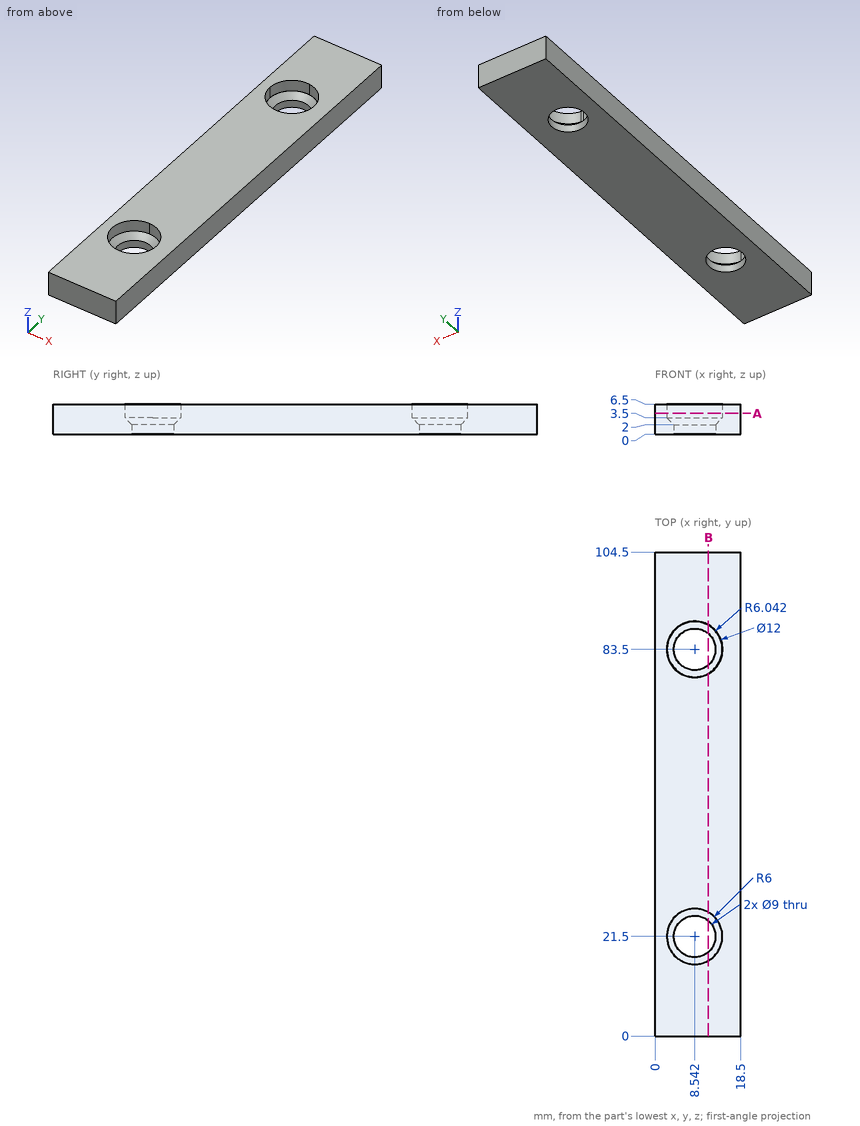
Could you check a few things on this drawing? It's one solid part, dimensions in mm from its lowest x, y, z. Round coordinates to 2 decimals unless told otherwise and drop trailing zeros. Write each loop counter-clockwise with the first axis right and the second up, starting at its lowest first coordinate (ties: lowest second). Pieces come first, ordered by that corner, then holes. Notation, with made-up numbers: M -31,59 L 24,59 A12 ccw 24,66 Z; hole C -12.75,-16 d5. An arc over 180 degrees is marked long. Answer as CSV lines item,"result". Start each with the question number.
1. I need wall thicknesses on probe 1 along Y at (x, z) = (8, 0.75); probe 2 along Y at (x, z) = (5.25, 0.75); probe 3 along X at (y, z) = (21.5, 0.9). Which ranges of each line are inside material? Lowest first, please.
2. Suppose I cut it at A-A on z = 4.5. Write out the boundary of the cut face in (x, y).
3. Suppose I cut it at B-B on x = 11.5. Count the separate pieces of the cut face and the enclosed holes in it, then the cut area to 3 significant figures.
Check result:
1,probe 1,"y = 0 to 17.03, 25.97 to 79.03, 87.97 to 104.5"
1,probe 2,"y = 0 to 18.43, 24.57 to 80.43, 86.57 to 104.5"
1,probe 3,"x = 0 to 4.04, 13.04 to 18.5"
2,outline,"M 0,0 L 18.5,0 L 18.5,104.5 L 0,104.5 Z; hole C 8.54,83.5 d12.08; hole C 8.54,21.5 d12"
3,separate pieces,"3"
3,enclosed holes,"0"
3,area,"563 mm2"
